The drawing under review shows one solid part. Ordinate dimensions are in mm from its lowest x, y, z. A direction names the side the tool comes from. Give positions to 0.01 mm unless a question says otherwise; leave off trailing zeros. Order: outer loops, then holes, each group sorted by start corner. A loop starts at its lowest first (then second) coordinate and runs counter-clockwise, first axis right, second up. Notation, with made-up numbers: (64.5, 48.25) - (84.5, 48.25) arc R5 ccw to (84.5, 56.25) - close; hole circle Ø5 at (46, 6). An arc over 180 degrees is marked (long way). Use CSV: the item, a comma, the result in double quotes. Start each with the question number.
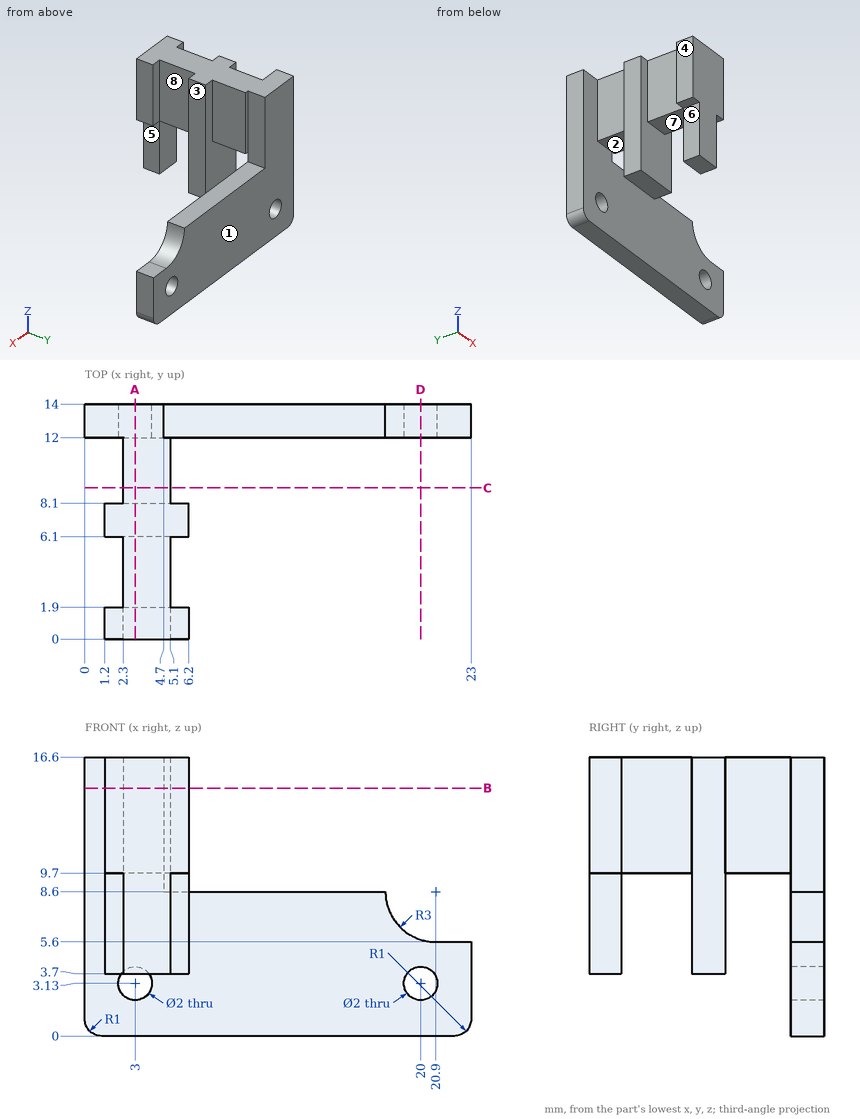
1. Mouldability with a two-part tool opening along Y and no side actions: class the marked faces 1, 2 and 3 as pulls with the +Y half, pulls with the -Y half, needs draft (parallel to the pull), parting line crosses it, or undercut.
2. Consider section C-C (y = 9). Give the boundary of the cut face in (x, z).
3. Tool access review of the marked faces 4, 5, 6, 7 and 8: name each direction out of +Z, -Z, +X, -X, +Y, -Y from which nothing blocks a thin tool from reaching the whole face with its end or side.
4. To check wall thickness, follow L1, parallel to Y at x = 2, z = 11.5; L2, parallel to X at y = 13, z = 2.75 (1 decimal); L3, parallel to Z at x = 3, y = 13.3. State the ranges of each line that lie inside material, in increasing order. Write a range as [from, to].
5. Consider section A-A (x = 3). Give the boundary of the cut face in (y, z).
6. Consider section D-D (x = 20). Give the boundary of the cut face in (y, z).
7. Consider section B-B (z = 14.75). Give the boundary of the cut face in (x, y).
8. Clearance check with flat-ended pins moving along their axes: pin 1 (2 mm diameter, centred on y = 9.5, z = 5.5, fed in from -X); pin 2 (1.6 mm diameter, centred on x = 22, y = 13, fed in from +Z); pin 3 (2 mm diameter, centred on y = 0.5, z = 14, fed in from +X); pin 4 (3 mm diameter, centred on y = 5.5, z = 2.5, fed in from -X). State where each tip first meets the part, or that it passes through.
Answers follow:
1,face 1,"pulls with the +Y half"
1,face 2,"undercut"
1,face 3,"needs draft"
2,outline,"(2.3, 9.7) - (5.1, 9.7) - (5.1, 16.6) - (2.3, 16.6) - close"
3,face 4,"+Z, -Z, -X, -Y"
3,face 5,"-Z, +X, -Y"
3,face 6,"-Z, -X, -Y"
3,face 7,"-Z, +X, -X"
3,face 8,"+Z, -Z, +X"
4,L1,"y = [0, 1.9], [6.1, 8.1], [12, 14]"
4,L2,"x = [0, 2.1], [3.9, 19.1], [20.9, 23]"
4,L3,"z = [0, 2.13], [4.13, 16.6]"
5,outline,"(0, 3.7) - (1.9, 3.7) - (1.9, 9.7) - (6.1, 9.7) - (6.1, 3.7) - (8.1, 3.7) - (8.1, 9.7) - (12, 9.7) - (12, 4.13) - (14, 4.13) - (14, 16.6) - (0, 16.6) - close; (12, 0) - (14, 0) - (14, 2.13) - (12, 2.13) - close"
6,outline,"(12, 0) - (14, 0) - (14, 2.13) - (12, 2.13) - close; (12, 4.13) - (14, 4.13) - (14, 5.74) - (12, 5.74) - close"
7,outline,"(0, 12) - (2.3, 12) - (2.3, 8.1) - (1.2, 8.1) - (1.2, 6.1) - (2.3, 6.1) - (2.3, 1.9) - (1.2, 1.9) - (1.2, 0) - (6.2, 0) - (6.2, 1.9) - (5.1, 1.9) - (5.1, 6.1) - (6.2, 6.1) - (6.2, 8.1) - (5.1, 8.1) - (5.1, 12) - (4.7, 12) - (4.7, 14) - (0, 14) - close"
8,pin 1,"passes through"
8,pin 2,"stops at z = 5.6"
8,pin 3,"stops at x = 6.2"
8,pin 4,"stops at x = 1.2"
